Part model, mm, in its own coordinate system. Coordinates: 2 decimals unless noted, no trailing zeros. Loops run counter-clockwise (first coordinate to the right, second up) from the corner with the lowest first, then second, coordinate; pieces in that order, holes last. Notation, with made-up numbers: (-17, 34.5) -> (22, 34.5) arc R17 cw to (22, 51.5) -> close; hole circle Ø10 at (-7.75, 47.25). An arc over 180 degrees is marked (long way). One line per item, written item: value. Start each with the question number.
from build123d import *

# Parameters (mm, degrees)
BOSS_EXTRUDE1_DEPTH        = 101.6
TAP_DRILL_FOR_10_24_TAP1_D = 3.7973
SKETCH6_R                  = 2.5527
CUT_EXTRUDE1_DEPTH         = 103.652877862


with BuildPart() as part:
    # Sketch1 → Boss-Extrude1 (new body)
    with BuildSketch(Plane(origin=(0, 0, 0), x_dir=(1, 0, 0), z_dir=(0, 1, 0))):
        Polygon((7.332348419, 0), (3.666174209, 6.35), (-3.666174209, 6.35), (-7.332348419, 0), (-3.666174209, -6.35), (3.666174209, -6.35), align=None)
    extrude(amount=BOSS_EXTRUDE1_DEPTH)

    # Tap Drill for #10-24 Tap1 (through all)
    with Locations(Plane.XY.offset(6.35)):
        with Locations((0, 95.25), (0, 6.35)):
            Hole(TAP_DRILL_FOR_10_24_TAP1_D / 2)

    # Sketch6 → Cut-Extrude1 (cut, through all)
    with BuildSketch(Plane.XY.offset(6.35)):
        with Locations((0, 31.75)):
            Circle(SKETCH6_R)
        with Locations((0, 69.85)):
            Circle(SKETCH6_R)
    extrude(amount=-CUT_EXTRUDE1_DEPTH, mode=Mode.SUBTRACT)


solid = part.part
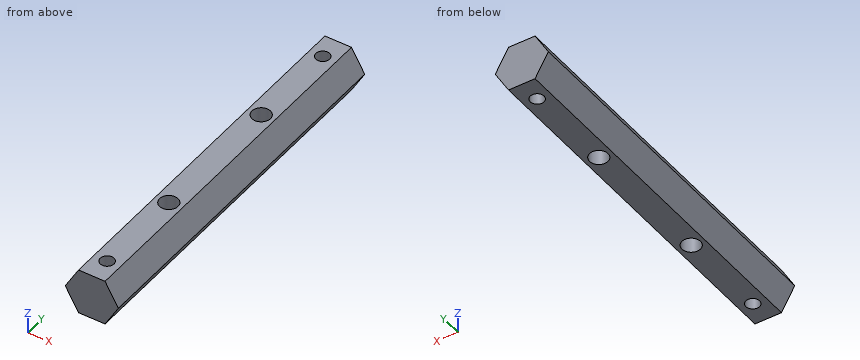
1) Pin check, flat tips, straight feed: pin 1 Ø2 at (x, z) = (-0.5, 2) entering from -Y; pin 2 Ø4 at (y, z) = (11.5, -2.5) entering from +X; pin 3 Ø1 at (y, z) = (72, 4) entering from -X. Stop position of each tip, or through.
2) Slice it at C-C (z = 1.75). Give the cut face in (x, y).
3) Slice it at B-B (x = 0). Give the cut face in (y, z), then the cut area to 3 significant figures.
4) Slice it at A-A (y = 6.35). Give the cut face in (x, z).
5) Probe line 1 (Y direction, x = 0, z = 1.75); line 2 (X direction, y = 95.25, z = 0); line 3 (X direction, y = 95.25, z = -1.25). List the from-to ranges inside material, lowest first. Write a range as from..to.
6) Slice it at D-D (y = 31.75). Give the cut face in (x, z), then the cut area to 3 significant figures.
Check sheet entries:
1. pin 1: stops at y = 0
1. pin 2: stops at x = 7.04
1. pin 3: stops at x = -5.31
2. outline: (-6.32, 0) -> (6.32, 0) -> (6.32, 101.6) -> (-6.32, 101.6) -> close; hole circle Ø5.11 at (0, 31.75); hole circle Ø5.11 at (0, 69.85); hole circle Ø3.8 at (0, 6.35); hole circle Ø3.8 at (0, 95.25)
3. outline: (0, -6.35) -> (4.45, -6.35) -> (4.45, 6.35) -> (0, 6.35) -> close; (8.25, -6.35) -> (29.2, -6.35) -> (29.2, 6.35) -> (8.25, 6.35) -> close; (34.3, -6.35) -> (67.3, -6.35) -> (67.3, 6.35) -> (34.3, 6.35) -> close; (72.4, -6.35) -> (93.35, -6.35) -> (93.35, 6.35) -> (72.4, 6.35) -> close; (97.15, -6.35) -> (101.6, -6.35) -> (101.6, 6.35) -> (97.15, 6.35) -> close
3. area: 1,060 mm^2
4. outline: (-7.33, 0) -> (-3.67, -6.35) -> (-1.9, -6.35) -> (-1.9, 6.35) -> (-3.67, 6.35) -> close; (1.9, -6.35) -> (3.67, -6.35) -> (7.33, 0) -> (3.67, 6.35) -> (1.9, 6.35) -> close
5. line 1: y = 0..4.45, 8.25..29.2, 34.3..67.3, 72.4..93.35, 97.15..101.6
5. line 2: x = -7.33..-1.9, 1.9..7.33
5. line 3: x = -6.61..-1.9, 1.9..6.61
6. outline: (-7.33, 0) -> (-3.67, -6.35) -> (-2.55, -6.35) -> (-2.55, 6.35) -> (-3.67, 6.35) -> close; (2.55, -6.35) -> (3.67, -6.35) -> (7.33, 0) -> (3.67, 6.35) -> (2.55, 6.35) -> close
6. area: 74.8 mm^2
